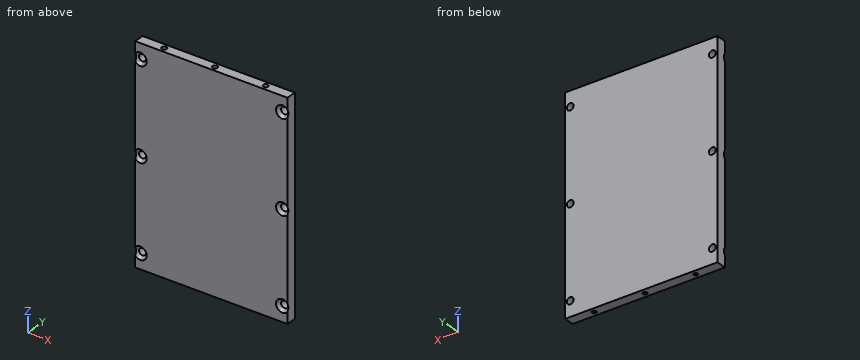
```python
from build123d import *

# Parameters (mm, degrees)
SKETCH_1_W                   = 75
SKETCH_1_H                   = 105
EXTRUDE_432_DEPTH            = 5
HOLE_WIZARD_M3_D             = 2.5
HOLE_WIZARD_M3_DEPTH         = 10
HOLE_WIZARD_M3_TIP           = 0.751075774
HOLE_WIZARD_M3_2_D           = 1.6
HOLE_WIZARD_M3_2_DEPTH       = 10
HOLE_WIZARD_M3_2_CSINK_D     = 2.05
HOLE_WIZARD_M3_2_CSINK_ANGLE = 90
HOLE_WIZARD_M3_2_TIP         = 0.480688495
HOLE_WIZARD_M3_3_D           = 3.4
HOLE_WIZARD_M3_3_CSINK_D     = 6.3
HOLE_WIZARD_M3_3_CSINK_ANGLE = 90


with BuildPart() as part:
    # Эскиз1 → Extrude 432 (new body)
    with BuildSketch(Plane(origin=(0, 0, 0), x_dir=(1, 0, 0), z_dir=(0, 1, 0))):
        with Locations((0, 31.5)):
            Rectangle(SKETCH_1_W, SKETCH_1_H)
    extrude(amount=EXTRUDE_432_DEPTH)

    # Hole Wizard M3
    with Locations(Plane.XY.offset(21)):
        with Locations((-25, 2.5), (0, 2.5), (25, 2.5)):
            Hole(HOLE_WIZARD_M3_D / 2, depth=HOLE_WIZARD_M3_DEPTH)
            with Locations((0, 0, -(HOLE_WIZARD_M3_DEPTH + HOLE_WIZARD_M3_TIP / 2))):  # 118° drill point
                Cone(0, HOLE_WIZARD_M3_D / 2, HOLE_WIZARD_M3_TIP, mode=Mode.SUBTRACT)

    # Hole Wizard M3 2
    with Locations(Plane(origin=(0, 0, -84), x_dir=(-1, 0, 0), z_dir=(0, 0, -1))):
        with Locations((-25, 2.5), (0, 2.5), (25, 2.5)):
            CounterSinkHole(HOLE_WIZARD_M3_2_D / 2, HOLE_WIZARD_M3_2_CSINK_D / 2, depth=HOLE_WIZARD_M3_2_DEPTH, counter_sink_angle=HOLE_WIZARD_M3_2_CSINK_ANGLE)
            with Locations((0, 0, -(HOLE_WIZARD_M3_2_DEPTH + HOLE_WIZARD_M3_2_TIP / 2))):  # 118° drill point
                Cone(0, HOLE_WIZARD_M3_2_D / 2, HOLE_WIZARD_M3_2_TIP, mode=Mode.SUBTRACT)

    # Hole Wizard M3 3 (through all)
    with Locations(Plane.XZ):
        with Locations((-35, -31.5), (35, -31.5), (35, -76.5), (35, 13.5), (-35, 13.5), (-35, -76.5)):
            CounterSinkHole(HOLE_WIZARD_M3_3_D / 2, HOLE_WIZARD_M3_3_CSINK_D / 2, counter_sink_angle=HOLE_WIZARD_M3_3_CSINK_ANGLE)


solid = part.part
```
Source: CAD feature listing. Evaluate the final solid. Frame: model axes, mm. Round coordinates to 2 decimals unless told otherwise and drop trailing zeros. Loops run counter-clockwise (first coordinate to the right, second up) from the corner with the lowest first, then second, coordinate; pieces in that order, holes last. Notation, with made-up numbers: M 88,61.5 L 102,61.5 A28 ccw 102,91.5 Z; hole C 44.5,78.5 d11. An arc over 180 degrees is marked long. Use a Markdown table: item, result. Add a question column.
1. Cut plane B-B, the plane x = -35. Output: boundary loops of the cut face in (y, z).
2. Contact query for flat-ended pins moving along their axis: pin 1 (4.5 mm diameter, centred on x = 35, z = -76.5, fed in from +Y); pin 2 (2 mm diameter, centred on x = 25, y = 2.5, fed in from -Z) (3 decimals); pin 3 (4.5 mm diameter, centred on x = 35, z = -31.5, fed in from -Y); pin 4 (1.8 mm diameter, centred on x = -25, y = 2.5, fed in from -Z) (3 decimals). Output: stop coordinate, or through.
3. Cut plane C-C, the plane z = -31.5. Output: boundary loops of the cut face in (x, y), and give its area (3 significant figures).
4. Ray query, line 1 along Z through (x, y) = (-35, 2.95); line 2 along X through (y, z) = (3.5, -31.5); line 3 along X through (y, z) = (2.5, -78.5). Return the intervals inside material, ascending. Write a range as [from, to].
5. Cut plane A-A, the plane z = -76.5. Output: boundary loops of the cut face in (x, y).
Solution:
| question | item | result |
|---|---|---|
| 1 | outline | M 0,-84 L 5,-84 L 5,-78.2 L 1.45,-78.2 L 0,-79.65 Z; M 0,-73.35 L 1.45,-74.8 L 5,-74.8 L 5,-33.2 L 1.45,-33.2 L 0,-34.65 Z; M 0,-28.35 L 1.45,-29.8 L 5,-29.8 L 5,11.8 L 1.45,11.8 L 0,10.35 Z; M 0,16.65 L 1.45,15.2 L 5,15.2 L 5,21 L 0,21 Z |
| 2 | pin 1 | stops at y = 5 |
| 2 | pin 2 | stops at z = -83.975 |
| 2 | pin 3 | stops at y = 0.9 |
| 2 | pin 4 | stops at z = -83.875 |
| 3 | outline | M -37.5,0.65 L -36.7,1.45 L -36.7,5 L -37.5,5 Z; M -33.3,1.45 L -31.85,0 L 31.85,0 L 33.3,1.45 L 33.3,5 L -33.3,5 Z; M 36.7,1.45 L 37.5,0.65 L 37.5,5 L 36.7,5 Z |
| 3 | area | 337 mm2 |
| 4 | line 1 | z = [-84, -78.2], [-74.8, -33.2], [-29.8, 11.8], [15.2, 21] |
| 4 | line 2 | x = [-37.5, -36.7], [-33.3, 33.3], [36.7, 37.5] |
| 4 | line 3 | x = [-37.5, -25.8], [-24.2, -0.8], [0.8, 24.2], [25.8, 37.5] |
| 5 | outline | M -37.5,0.65 L -36.7,1.45 L -36.7,5 L -37.5,5 Z; M -33.3,1.45 L -31.85,0 L 31.85,0 L 33.3,1.45 L 33.3,5 L -33.3,5 Z; M 36.7,1.45 L 37.5,0.65 L 37.5,5 L 36.7,5 Z; hole C -25,2.5 d1.6; hole C 0,2.5 d1.6; hole C 25,2.5 d1.6 |
